Build history of the part. All positions in model axes, mm. Give positions to 0.01 mm unless a question says otherwise; leave off trailing zeros. Write each loop counter-clockwise with the first axis right and the second up, starting at its lowest first coordinate (ties: lowest second). Pieces come first, ordered by that corner, then holes.
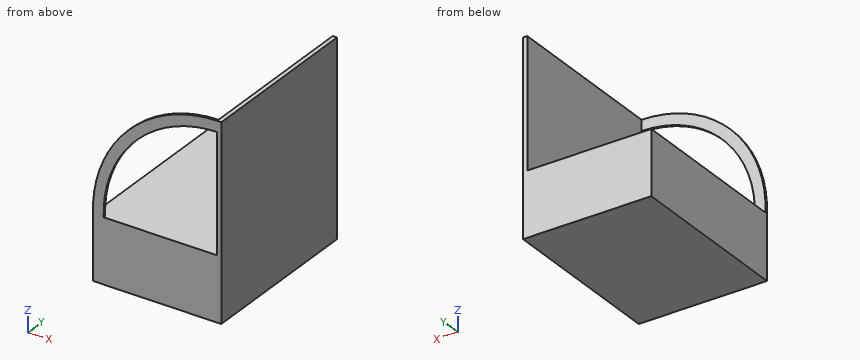
Autodesk Inventor part; units mm, degrees
ref_plane "YZ Plane" through (0, 0, 0) normal (1, 0, 0) x (0, 1, 0)
ref_plane "XZ Plane" through (0, 0, 0) normal (0, 1, 0) x (-1, 0, 0)
ref_plane "XY Plane" through (0, 0, 0) normal (0, 0, 1) x (1, 0, 0)
sketch "Sketch1" plane through (0, 0, 0) normal (0, 1, 0) x (-1, 0, 0)
  line L0 (0, 0) -> (-600, 0)
  line L1 (-600, 0) -> (-600, 300)
  line L2 (-600, 300) -> (0, 300)
  line L3 (0, 300) -> (0, 0)
  line L4 (0, 300) -> (-20, 300)
  line L5 (-600, 300) -> (-580, 300)
  line L6 (-580, 300) -> (-580, 900)
  line L7 (-580, 900) -> (-600, 900)
  line L8 (-600, 900) -> (-600, 300)
  dimension "d0" = 600
  dimension "d1" = 300
  dimension "d9" = 600
  dimension "d10" = 20
extrude "Extrusion1" add sketch "Sketch1" along normal blind 800
sketch "Sketch3" plane through (0, 0, 0) normal (0, 1, 0) x (-1, 0, 0)
  line L0 (0, 300) -> (-580, 300)
  line L1 (-580, 300) -> (-580, 900)
  line L2 (-580, 900) -> (-600, 900)
  line L3 (-600, 900) -> (-600, 0)
  line L4 (-600, 0) -> (0, 0)
  line L5 (0, 0) -> (0, 300)
  arc A0 (0, 300) -> (-580, 900) centre (-580, 319.6667) ccw
  arc A1 (-50.0314, 300) -> (-580, 850) centre (-580, 319.6667) ccw
  dimension "d11" = 50
extrude "Extrusion3" add sketch "Sketch3" along normal blind 10 contours L0 A1 L1 A0
equation "\"d9\" = d0"
properties part number "Electrical box 1"
1. Saw through at A-A on z = 562. Give the cut face in (x, y), plus the area to 3 significant figures.
2. Saw through at B-B on x = 93. Give the cut face in (y, z).
3. Saw through at C-C on y = 444. Give the cut face in (x, z).
4. Drill centre lines: line 1 along Z through (x, y) = (176.5, 85.5); line 2 along X through (y, z) = (331.5, 317); line 3 along X through (y, z) = (154, 65). Where is each one in solid material? Low to high.
5. Drop a flat-ended pin along its axis: pin 1 (5 mm diameter, centred on x = 349.5, y = 589, fed in from +Z). Give the stop position or say it passes through.
Outcome:
1. outline: (52.68, 0) - (108.27, 0) - (108.27, 10) - (52.68, 10) - close; (580, 0) - (600, 0) - (600, 800) - (580, 800) - close
1. area: 16,600 mm2
2. outline: (0, 0) - (800, 0) - (800, 300) - (0, 300) - close; (0, 529.63) - (10, 529.63) - (10, 635.29) - (0, 635.29) - close
3. outline: (0, 0) - (600, 0) - (600, 900) - (580, 900) - (580, 300) - (0, 300) - close
4. line 1: z = 0 to 300
4. line 2: x = 580 to 600
4. line 3: x = 0 to 600
5. pin 1: stops at z = 300
